Check sheet for the drawn part. Datum: minimum x, y, z corner. Units: mm. Round coordinates to 2 decimals unless told otherwise and drop trailing zeros. Order: outer loops, then holes, each group sorted by start corner. A loop starts at its lowest first (then second) coordinate and runs counter-clockwise, first axis right, second up.
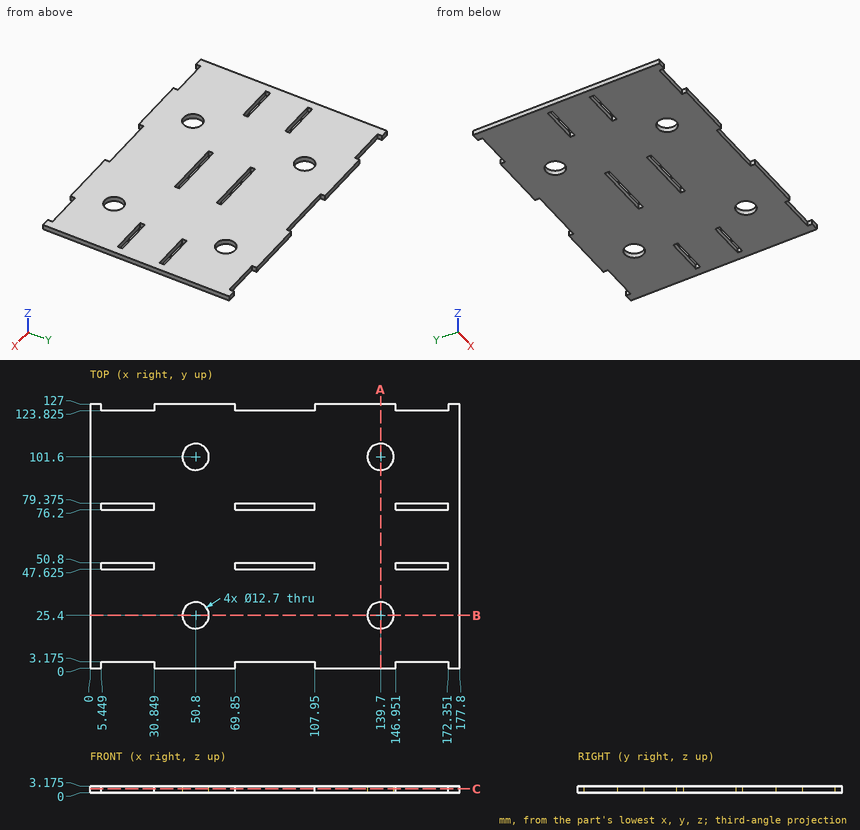
(1) Material ranges on line 1 (Y direction, x = 90.5, z = 1.05) (3 decimals); line 2 (X direction, y = 50, z = 0.95); line 3 (Y direction, x = 139.7, z = 1.25), recorded low to high.
Returned:
line 1: y = 3.175 to 47.625, 50.8 to 76.2, 79.375 to 123.825
line 2: x = 0 to 5.45, 30.85 to 69.85, 107.95 to 146.95, 172.35 to 177.8
line 3: y = 0 to 19.05, 31.75 to 95.25, 107.95 to 127
(2) Sectioned sample at C-C, the plane z = 1.9. Give the number of separate pieces and of enclosed holes in the cut face, and give its area (3 significant figures).
Returned:
separate pieces: 1
enclosed holes: 10
area: 20,900 mm2
(3) Sectioned sample at B-B, the plane y = 25.4. Record the cut outline in (x, z) (3 decimals).
Returned:
outline: (0, 0) - (44.45, 0) - (44.45, 3.175) - (0, 3.175) - close; (57.15, 0) - (133.35, 0) - (133.35, 3.175) - (57.15, 3.175) - close; (146.05, 0) - (177.8, 0) - (177.8, 3.175) - (146.05, 3.175) - close
(4) Depth check by flat-ended pin: P1, Ø1.6, axis at x = 87, z = 1.5, coming from the +Y side (3 decimals); P2, Ø1, axis at y = 78, z = 1, coming from the -X side; P3, Ø1.6, axis at x = 92.5, z = 1.5, coming from the -Y side (3 decimals). Enter the tip coordinate at first touch or a pass-through.
Returned:
P1: stops at y = 123.825
P2: stops at x = 0
P3: stops at y = 3.175
(5) Sectioned sample at A-A, the plane x = 139.7. Record the cut outline in (y, z) (3 decimals).
Returned:
outline: (0, 0) - (19.05, 0) - (19.05, 3.175) - (0, 3.175) - close; (31.75, 0) - (95.25, 0) - (95.25, 3.175) - (31.75, 3.175) - close; (107.95, 0) - (127, 0) - (127, 3.175) - (107.95, 3.175) - close
